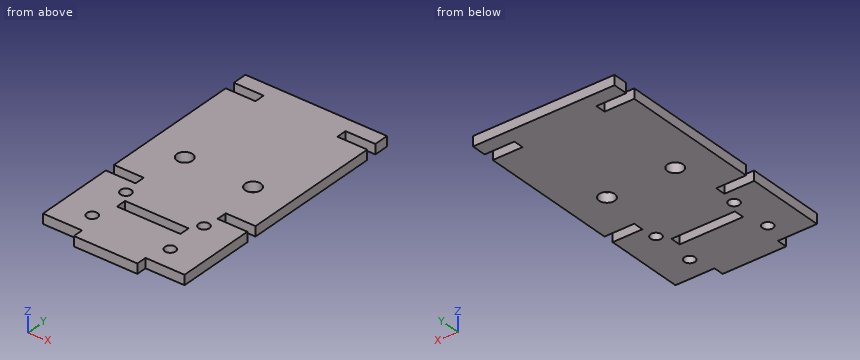
from build123d import *

# Parameters (mm, degrees)
SKETCH_1_W          = 8
SKETCH_1_H          = 2.1
SKETCH_1_W_2        = 13
EXTRUDE_1_DEPTH     = 2
SKETCH_2_W          = 6.1
SKETCH_2_H          = 2.1
CUT_EXTRUDE_1_DEPTH = 2
SKETCH_3_W          = 16.8
SKETCH_3_H          = 2.1
EXTRUDE_2_DEPTH     = 2
SKETCH_4_R          = 1.6
CUT_EXTRUDE_2_DEPTH = 2
SKETCH_5_R          = 1.1
CUT_EXTRUDE_5_DEPTH = 10
SKETCH_6_R          = 1.1
CUT_EXTRUDE_6_DEPTH = 10
EXTRUDE_3_DEPTH     = 2


with BuildPart() as part:
    # 草图1 → 凸台-拉伸1 (new body)
    with BuildSketch(Plane.XY):
        Polygon((-12.242924528, 31.300471698), (-12.242924528, -4.699528302), (-4.242924528, -4.699528302), (8.757075472, -4.699528302), (16.757075472, -4.699528302), (16.757075472, 31.300471698), align=None)
        Polygon((-12.242924528, -6.799528302), (-12.242924528, -15.799528302), (-4.242924528, -15.799528302), (8.757075472, -15.799528302), (16.757075472, -15.799528302), (16.757075472, -6.799528302), (8.757075472, -6.799528302), (-4.242924528, -6.799528302), align=None)
        with Locations((12.757075472, -5.749528302)):
            Rectangle(SKETCH_1_W, SKETCH_1_H)
        with Locations((-8.242924528, -5.749528302)):
            Rectangle(SKETCH_1_W, SKETCH_1_H)
        with Locations((2.257075472, -16.849528302)):
            Rectangle(SKETCH_1_W_2, SKETCH_1_H)
    extrude(amount=EXTRUDE_1_DEPTH)

    # 草图2 → 切除-拉伸1 (cut)
    with BuildSketch(Plane.XY.offset(2)):
        with Locations((13.707075472, 1.450471698)):
            Rectangle(SKETCH_2_W, SKETCH_2_H)
        with Locations((-9.192924528, 1.450471698)):
            Rectangle(SKETCH_2_W, SKETCH_2_H)
    extrude(amount=-CUT_EXTRUDE_1_DEPTH, mode=Mode.SUBTRACT)

    # 草图3 → 凸台-拉伸2 (add)
    with BuildSketch(Plane.XY.offset(2)):
        with Locations((2.257075472, 32.350471698)):
            Rectangle(SKETCH_3_W, SKETCH_3_H)
    extrude(amount=-EXTRUDE_2_DEPTH)

    # 草图4 → 切除-拉伸2 (cut)
    with BuildSketch(Plane.XY.offset(2)):
        with Locations((-4.742924528, 11.300471698)):
            Circle(SKETCH_4_R)
        with Locations(Location((9.257075472, 11.300471698, 0), (0, 0, 180))):
            Circle(SKETCH_4_R)
    extrude(amount=-CUT_EXTRUDE_2_DEPTH, mode=Mode.SUBTRACT)

    # 草图5 → 切除-拉伸5 (cut)
    with BuildSketch(Plane(origin=(0, 0, 0), x_dir=(-1, 0, 0), z_dir=(0, 0, -1))):
        with Locations((-10.257075472, -2.599528302)):
            Circle(SKETCH_5_R)
        with Locations((5.742924528, -2.599528302)):
            Circle(SKETCH_5_R)
    extrude(amount=-CUT_EXTRUDE_5_DEPTH, mode=Mode.SUBTRACT)

    # 草图6 → 切除-拉伸6 (cut)
    with BuildSketch(Plane.XY.offset(2)):
        with Locations((10.257075472, -11.299528302)):
            Circle(SKETCH_6_R)
        with Locations((-5.742924528, -11.299528302)):
            Circle(SKETCH_6_R)
    extrude(amount=-CUT_EXTRUDE_6_DEPTH, mode=Mode.SUBTRACT)

    # 草图7 → 凸台-拉伸3 (add)
    with BuildSketch(Plane.XY.offset(2)):
        Polygon((-6.142924528, 33.400471698), (-12.242924528, 33.400471698), (-12.242924528, 36.400471698), (16.757075472, 36.400471698), (16.757075472, 33.400471698), align=None)
    extrude(amount=-EXTRUDE_3_DEPTH)


solid = part.part
Geometry check sheet. Reference: the model listing, model coordinates, mm. Round coordinates to 2 decimals unless told otherwise and drop trailing zeros. Order: outer loops, then holes, each group sorted by start corner. A loop starts at its lowest first (then second) coordinate and runs counter-clockwise, first axis right, second up. Notation, with made-up numbers: (46.25, 23.25) - (89.25, 23.25) arc R24 cw to (89.25, 39.25) - close; hole circle Ø10 at (74.5, 46.25). An arc over 180 degrees is marked (long way). One line per question, with ' | ' between items. Start each with the question number.
(1) Sectioned sample at A-A on x = 5.25. Record the cut outline in (y, z), and give its area (3 significant figures).
(2) Sectioned sample at C-C on z = 1.3. Count the separate pieces of the cut face and the enclosed holes in it, and give its area (3 significant figures).
(3) Thickness scan on L1, parallel to Y at x = 14.25, z = 1; L2, parallel to Y at x = 1, z = 1.3; L3, parallel to X at y = 10.5, z = 1.3. Record the ranges inside material, lowest first. Write a range as [from, to].
(4) Sectioned sample at B-B on x = -9. Record the cut outline in (y, z), and give its area (3 significant figures).
(5) Sectioned sample at D-D on x = 9.75. Record the cut outline in (y, z).
(6) Depth check by flat-ended pin: pin 1 Ø0.6 at (x, z) = (-8.5, 1) entering from -Y. Enter the tip coordinate at first touch or a pass-through.
Conclusion:
1) outline: (-17.9, 0) - (-6.8, 0) - (-6.8, 2) - (-17.9, 2) - close; (-4.7, 0) - (36.4, 0) - (36.4, 2) - (-4.7, 2) - close | area: 104 mm2
2) separate pieces: 1 | enclosed holes: 7 | area: 1,430 mm2
3) L1: y = [-15.8, 0.4], [2.5, 31.3], [33.4, 36.4] | L2: y = [-17.9, -6.8], [-4.7, 36.4] | L3: x = [-12.24, -6.13], [-3.36, 7.87], [10.64, 16.76]
4) outline: (-15.8, 0) - (0.4, 0) - (0.4, 2) - (-15.8, 2) - close; (2.5, 0) - (31.3, 0) - (31.3, 2) - (2.5, 2) - close; (33.4, 0) - (36.4, 0) - (36.4, 2) - (33.4, 2) - close | area: 96.0 mm2
5) outline: (-15.8, 0) - (-12.28, 0) - (-12.28, 2) - (-15.8, 2) - close; (-10.32, 0) - (-3.58, 0) - (-3.58, 2) - (-10.32, 2) - close; (-1.62, 0) - (9.78, 0) - (9.78, 2) - (-1.62, 2) - close; (12.82, 0) - (36.4, 0) - (36.4, 2) - (12.82, 2) - close
6) pin 1: stops at y = -15.8
